Answer from the drawing. Dimensions are ordinates in mm from the lowest x, y and z of the part. A direction names the side the tool comes from. Give positions to 0.01 mm unless a question says otherwise; leave off trailing zeros. Order: outer loops, then holes, each group sorted by start corner. A loop starts at its lowest first (then second) coordinate and runs counter-clockwise, first axis right, second up. Notation, with made-up numbers: M -10.5,38.25 L -1.5,38.25 A25 cw -1.5,70.25 Z; hole C 50,56.5 d2. An arc over 180 degrees is marked long. One line per item, written item: value.
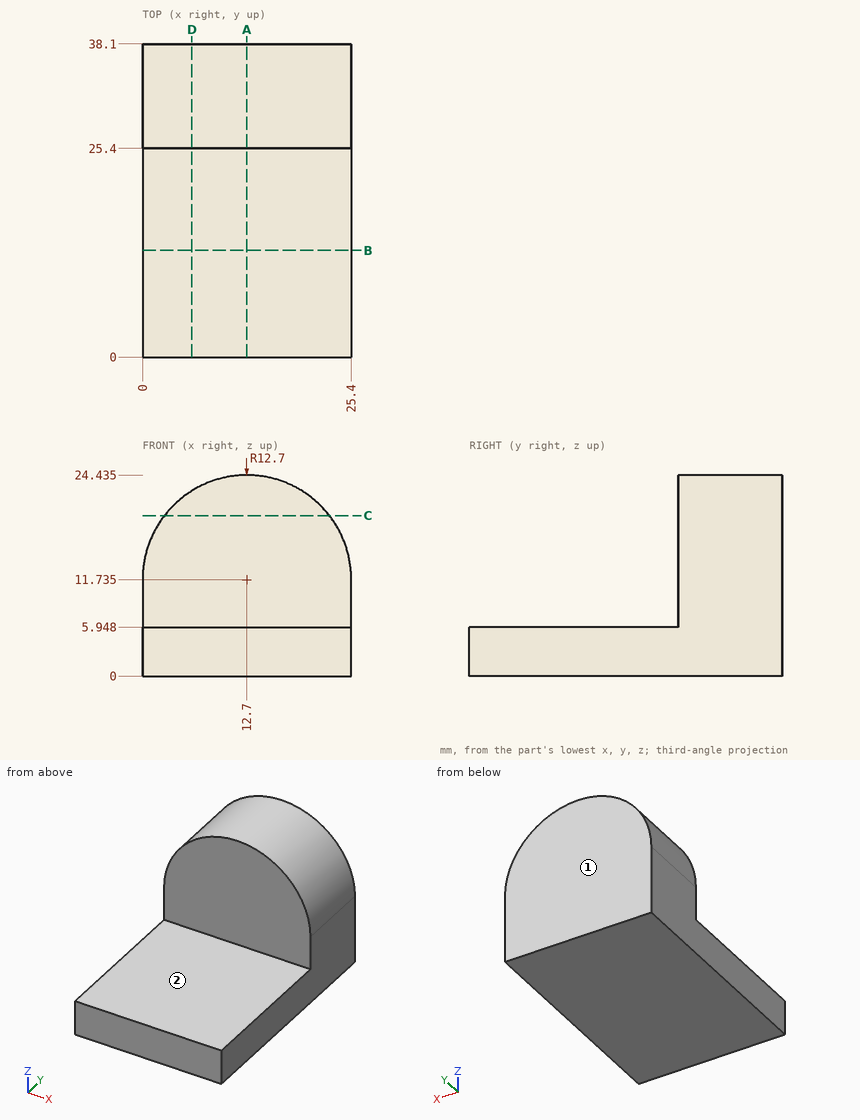
(1) Which of the six approach directions +Z, -Z, +X, -X, +Y, -Y give full straight-line access (tool end or side, diameter ignored) to the marked faces 1 and 2?
Findings:
face 1: +Z, -Z, +X, -X, +Y
face 2: +Z, +X, -X, -Y
(2) Find the intervals of material crossed by probe 1 along Z at (x, y) = (8.5, 9); probe 2 along Y at (x, z) = (3, 10); probe 3 along Z at (x, y) = (20.25, 28.5), in increasing order. Write a range as from..to.
Findings:
probe 1: z = 0..5.95
probe 2: y = 25.4..38.1
probe 3: z = 0..21.95
(3) Given P1, Ø1.5, axis at x = 12, y = 29, coming from the +Z side (1 decimal); P2, Ø12.5, axis at x = 12, y = 11, coming from the +Z side, each flat-ended and moving along its own axis, determine where each tip first touches the part or whether it passes through.
Findings:
P1: stops at z = 24.4
P2: stops at z = 5.95
(4) Section B-B, the plane y = 13 is taken. Give the vertices of the cut face in (x, z), then the cut area to 3 significant figures.
Findings:
outline: M 0,0 L 25.4,0 L 25.4,5.95 L 0,5.95 Z
area: 151 mm^2
(5) Section C-C, the plane z = 19.5 is taken. Give the vertices of the cut face in (x, y), then the cut area to 3 significant figures.
Findings:
outline: M 2.65,25.4 L 22.75,25.4 L 22.75,38.1 L 2.65,38.1 Z
area: 255 mm^2
(6) Section D-D, the plane x = 6 is taken. Give the vertices of the cut face in (y, z) (1 decimal).
Findings:
outline: M 0,0 L 38.1,0 L 38.1,22.5 L 25.4,22.5 L 25.4,5.9 L 0,5.9 Z
(7) Section A-A, the plane x = 12.7 is taken. Give the vertices of the cut face in (y, z) (1 decimal).
Findings:
outline: M 0,0 L 38.1,0 L 38.1,24.4 L 25.4,24.4 L 25.4,5.9 L 0,5.9 Z
